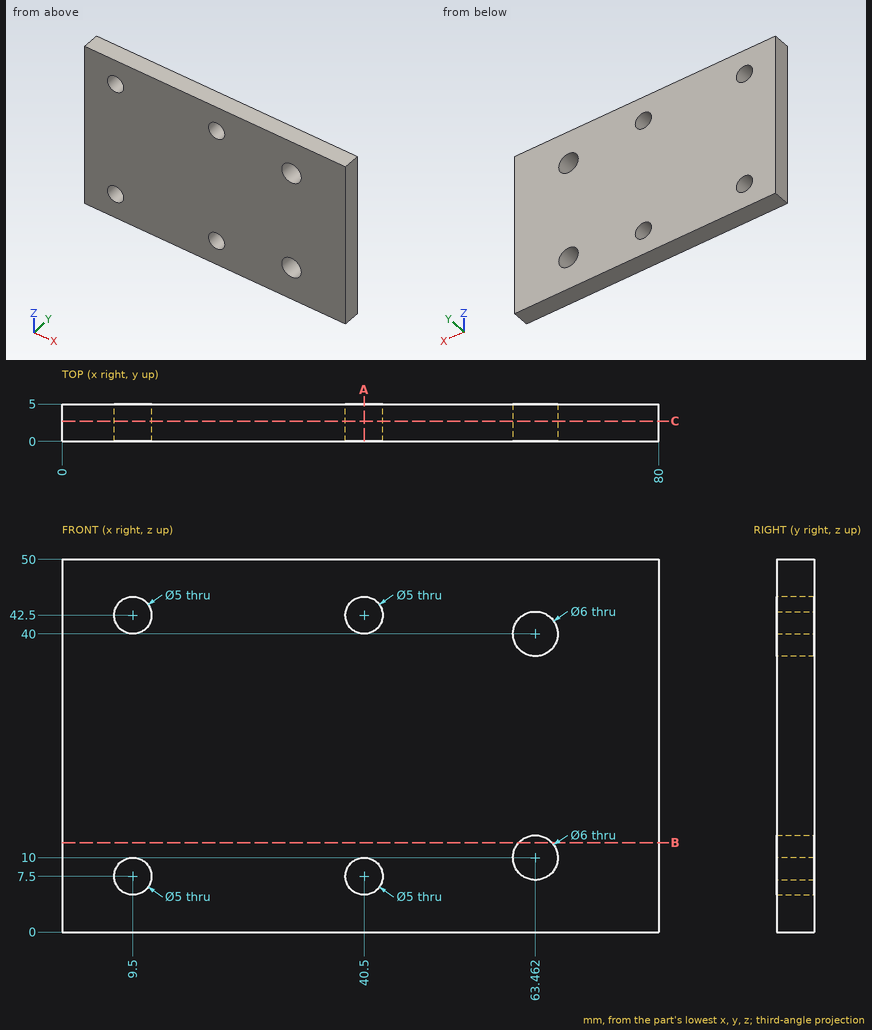
Answer from the drawing. Dimensions are ordinates in mm from the lowest x, y and z of the part. Coordinates: 2 decimals unless noted, no trailing zeros. Write each loop counter-clockwise with the first axis right and the second up, starting at its lowest first coordinate (ties: lowest second). Pieces come first, ordered by that corner, then holes. Notation, with made-up numbers: (11.25, 8.5) - (23.25, 8.5) arc R26 cw to (23.25, 45.5) - close; hole circle Ø6 at (38.5, -8). An arc over 180 degrees is marked (long way). Return JSON: item names as keys, results as strings.
1. The part is cut by section B-B on z = 12. Determine the outline of the cut face in (x, y) (1 decimal).
Final values:
{"outline": "(0, 0) - (61.2, 0) - (61.2, 5) - (0, 5) - close; (65.7, 0) - (80, 0) - (80, 5) - (65.7, 5) - close"}
2. The part is cut by section C-C on y = 2.7. Determine the outline of the cut face in (x, z).
Final values:
{"outline": "(0, 0) - (80, 0) - (80, 50) - (0, 50) - close; hole circle Ø5 at (9.5, 7.5); hole circle Ø5 at (9.5, 42.5); hole circle Ø5 at (40.5, 7.5); hole circle Ø5 at (40.5, 42.5); hole circle Ø6 at (63.46, 10); hole circle Ø6 at (63.46, 40)"}
3. The part is cut by section A-A on x = 40.5. Determine the outline of the cut face in (y, z), then the cut area to 3 significant figures.
Final values:
{"outline": "(0, 0) - (5, 0) - (5, 5) - (0, 5) - close; (0, 10) - (5, 10) - (5, 40) - (0, 40) - close; (0, 45) - (5, 45) - (5, 50) - (0, 50) - close", "area": "200 mm^2"}
4. Consider line 1 along X through (y, z) = (1.3, 42.5) (1 decimal); line 2 along Z through (x, y) = (39, 2.95); line 3 along Z through (x, y) = (39.5, 1.05). Determine where each line is inside the solid, lowest interval first.
Final values:
{"line 1": "0 to 7, 12 to 38, 43 to 61.8, 65.1 to 80", "line 2": "0 to 5.5, 9.5 to 40.5, 44.5 to 50", "line 3": "0 to 5.21, 9.79 to 40.21, 44.79 to 50"}
